The listing builds one solid part. Answer for the finished solid, in the listing's coordinates (mm). A direction names the side the tool comes from. Give positions to 0.01 mm unless a question says otherwise; leave off trailing zeros. Loops run counter-clockwise (first coordinate to the right, second up) from the corner with the lowest first, then second, coordinate; pieces in that order, holes last. Notation, with made-up numbers: (10.5, -4.75) - (57.5, -4.75) arc R18 cw to (57.5, 29.25) - close; hole circle Ø4 at (54, 77.5). An arc over 180 degrees is marked (long way). Write each question's results on one line, items separated by ' | '.
from build123d import *

# Parameters (mm, degrees)
F0_W       = 127
F0_H       = 127
F1_DEPTH   = 50.8
F2_W       = 19.05
F2_H       = 50.8
F2_H_2     = 127
F3_DEPTH   = 25.4
F3_FACE_W  = 50.8
F3_FACE_H  = 25.4
F3_FACE1_W = 127
F3_FACE1_H = 25.4
F5_T       = -2.54


with BuildPart() as f1:
    # F0 (on Top) → F1 (new body)
    with BuildSketch(Plane.XY):
        with Locations((63.5, 63.5)):
            Rectangle(F0_W, F0_H)
    extrude(amount=F1_DEPTH)

    # F2 (on face) → F3 (join)
    with BuildSketch(Plane.XY.offset(50.8)):
        with Locations((9.525, 63.5)):
            Rectangle(F2_W, F2_H)
        with Locations((117.475, 63.5)):
            Rectangle(F2_W, F2_H_2)
    extrude(amount=F3_DEPTH)

    # F3_face (on face) → F4 section 0
    with BuildSketch(Plane(origin=(19.05, 63.5, 63.5), x_dir=(0, 1, 0), z_dir=(1, 0, 0))):
        Rectangle(F3_FACE_W, F3_FACE_H)
    # F3_face1 (on face) → F4 section 1
    with BuildSketch(Plane(origin=(107.95, 63.5, 63.5), x_dir=(0, -1, 0), z_dir=(-1, 0, 0))):
        Rectangle(F3_FACE1_W, F3_FACE1_H)
    loft()

    # F5
    f5_openings = [f1.faces().sort_by_distance(p)[0] for p in [
        (74.884643, 63.5, 76.2),
    ]]
    offset(amount=F5_T, openings=f5_openings, kind=Kind.INTERSECTION)


solid = f1.part
Item 1: A cutting plane is placed at A-A, the plane z = 40. Determine the outline of the cut face in (x, y), plus the area to 3 significant figures.
Values found:
outline: (0, 0) - (127, 0) - (127, 127) - (0, 127) - close; hole (2.54, 2.54) - (124.46, 2.54) - (124.46, 124.46) - (2.54, 124.46) - close | area: 1,260 mm²
Item 2: Find the intervals of material crossed by line 1 along Y through (x, z) = (58.5, 36.5); line 2 along Z through (x, y) = (40, 8), in increasing order. Write a range as [from, to].
Values found:
line 1: y = [0, 2.54], [124.46, 127] | line 2: z = [0, 2.54], [48.26, 50.8]
Item 3: A cutting plane is placed at D-D, the plane z = 58. Determine the outline of the cut face in (x, y).
Values found:
outline: (0, 38.1) - (19.05, 38.1) - (107.95, 0) - (127, 0) - (127, 127) - (107.95, 127) - (19.05, 88.9) - (0, 88.9) - close; hole (2.54, 40.64) - (19.57, 40.64) - (108.47, 2.54) - (124.46, 2.54) - (124.46, 124.46) - (108.47, 124.46) - (19.57, 86.36) - (2.54, 86.36) - close
Item 4: For faces 4 (the face through (124.46, 63, 39)), 5 (the face through (9, 38.1, 63)), 6 (the face through (63, 2.54, 31)), 7 (the face through (64.122, 108.217, 63.322)), determine the directions among +Z, -Z, +X, -X, +Y, -Y from which every point of the face is accessible in a straight line to the end or side of a thin tool.
Values found:
face 4: +Z | face 5: +Z, -X, -Y | face 6: none | face 7: +Z, -X, +Y
Item 5: A cutting plane is placed at C-C, the plane x = 85.5. Determine the outline of the cut face in (y, z), plus the area to 3 significant figures.
Values found:
outline: (0, 0) - (127, 0) - (127, 50.8) - (117.38, 50.8) - (117.38, 76.2) - (114.62, 76.2) - (114.62, 48.26) - (124.46, 48.26) - (124.46, 2.54) - (2.54, 2.54) - (2.54, 48.26) - (12.38, 48.26) - (12.38, 76.2) - (9.62, 76.2) - (9.62, 50.8) - (0, 50.8) - close | area: 758 mm²
Item 6: Flat-ended cylindrical pins translate along their axes: P1, Ø5.5, axis at x = 8.5, z = 58.5, coming from the -Y side; P2, Ø5, axis at x = 14, z = 60.5, coming from the +Y side; P3, Ø10, axis at y = 15.5, z = 66, coming from the -X side. Find the tip coordinate at first contact, or state that the pin passes through.
Values found:
P1: stops at y = 38.1 | P2: stops at y = 88.9 | P3: stops at x = 60.12
Item 7: For a pull along X with two mould halves and no side action, classify faces 1 (the face through (11, 86.36, 62)), 2 (the face through (0, 63, 29)), 3 (the face through (125, 69, 76.2)) as released by +X, released by -X, zero draft, split by the parting line, or undercut.
Values found:
face 1: undercut | face 2: released by -X | face 3: zero draft
Item 8: A cutting plane is placed at B-B, the plane y = 43. Determine the outline of the cut face in (x, z).
Values found:
outline: (0, 0) - (127, 0) - (127, 76.2) - (124.46, 76.2) - (124.46, 2.54) - (2.54, 2.54) - (2.54, 76.2) - (0, 76.2) - close
